```python
from build123d import *

# Parameters (mm, degrees)
SKETCH1_W           = 130
SKETCH1_H           = 180
BOSS_EXTRUDE1_DEPTH = 70
CUT_EXTRUDE1_DEPTH  = 131
FILLET2_R           = 4
SHELL1_T            = -2.5
SKETCH3_R           = 8
SKETCH3_W           = 60
SKETCH3_H           = 45
CUT_EXTRUDE2_DEPTH  = 10
CUT_EXTRUDE3_START  = -2.5
SKETCH4_W           = 69.3
SKETCH4_H           = 50
CUT_EXTRUDE3_DEPTH  = 1


with BuildPart() as part:
    # Sketch1 → Boss-Extrude1 (new body)
    with BuildSketch(Plane.XY):
        Rectangle(SKETCH1_W, SKETCH1_H)
    extrude(amount=BOSS_EXTRUDE1_DEPTH)

    # Sketch2 → Cut-Extrude1 (cut, through all)
    with BuildSketch(Plane.ZY.offset(65)):
        Polygon((70, -50), (25, -90), (70, -90), align=None)
    extrude(amount=-CUT_EXTRUDE1_DEPTH, mode=Mode.SUBTRACT)

    # Fillet2
    fillet2_edges = [part.edges().sort_by_distance(p)[0] for p in [
        (-65, 20, 70),
        (65, -90, 12.5),
        (-65, -90, 12.5),
        (0, -50, 70),
        (65, -70, 47.5),
        (0, -90, 25),
        (-65, -70, 47.5),
        (0, 90, 70),
        (65, 20, 70),
        (-65, 90, 35),
        (65, 90, 35),
    ]]
    fillet(fillet2_edges, radius=FILLET2_R)

    # Shell1
    shell1_openings = [part.faces().sort_by_distance(p)[0] for p in [
        (0, 0, 0),
    ]]
    offset(amount=SHELL1_T, openings=shell1_openings, kind=Kind.INTERSECTION)

    # Sketch3 → Cut-Extrude2 (cut)
    with BuildSketch(Plane(origin=(0, -62.689655172, 55.724137931), x_dir=(1, 0, 0), z_dir=(0, -0.747409319, 0.664363839))):
        with Locations((40.000108275, -9.586715238)):
            Circle(SKETCH3_R)
        with Locations((-11.005976929, -9.586715238)):
            Rectangle(SKETCH3_W, SKETCH3_H)
    extrude(amount=-CUT_EXTRUDE2_DEPTH, mode=Mode.SUBTRACT)

    # Sketch4 → Cut-Extrude3 (cut)
    with BuildSketch(Plane(origin=(0, -62.689655172, 55.724137931), x_dir=(1, 0, 0), z_dir=(0, -0.747409319, 0.664363839)).offset(CUT_EXTRUDE3_START)):
        with Locations((-8.85597671, -9.586715238)):
            Rectangle(SKETCH4_W, SKETCH4_H)
    extrude(amount=CUT_EXTRUDE3_DEPTH, mode=Mode.SUBTRACT)


solid = part.part
```
Geometry check sheet. Reference: the model listing, model coordinates, mm. A direction names the side the tool comes from. Coordinates: 2 decimals unless noted, no trailing zeros. Loops run counter-clockwise (first coordinate to the right, second up) from the corner with the lowest first, then second, coordinate; pieces in that order, holes last. Notation, with made-up numbers: (-30.75, 17.25) -> (-19.75, 17.25) arc R18 ccw to (-19.75, 44.25) -> close; hole circle Ø6 at (45, 84.5). An arc over 180 degrees is marked (long way). Put each result on its own line as item: value.
1) Cross-section at A-A on x = -13. Record the boundary of the cut face in (y, z), plus the area to 3 significant figures.
Result set:
outline: (-90, 0) -> (-87.5, 0) -> (-87.5, 23.48) arc R1.5 cw to (-87.12, 24.48) -> (-83.8, 28.21) -> (-84.55, 28.88) -> (-82.89, 30.75) -> (-84.01, 31.74) -> (-88.99, 26.14) arc R4 ccw to (-90, 23.48) -> close; (-54.11, 65.38) -> (-52.99, 64.38) -> (-51.33, 66.25) -> (-50.58, 65.58) -> (-49.32, 67) arc R1.5 cw to (-48.2, 67.5) -> (86, 67.5) arc R1.5 cw to (87.5, 66) -> (87.5, 0) -> (90, 0) -> (90, 66) arc R4 ccw to (86, 70) -> (-48.2, 70) arc R4 ccw to (-51.19, 68.66) -> close
area: 606 mm^2
2) Cross-section at B-B on y = -21. Record the boundary of the cut face in (x, z), plus the area to 3 significant figures.
Result set:
outline: (-65, 0) -> (-62.5, 0) -> (-62.5, 66) arc R1.5 cw to (-61, 67.5) -> (61, 67.5) arc R1.5 cw to (62.5, 66) -> (62.5, 0) -> (65, 0) -> (65, 66) arc R4 ccw to (61, 70) -> (-61, 70) arc R4 ccw to (-65, 66) -> close
area: 657 mm^2
3) Release check for a two-part mould opening along Y. For faces 3 (the flat face through (-1, 20, 70)), 4 (the cylindrical face through (0.854, 88.859, 68.797)), 5 (the flat face through (-43.506, -68, 47)) record: released by +Y, released by -Y, zero draft, split by the parting line, or undercut.
Result set:
face 3: zero draft
face 4: released by +Y
face 5: undercut
4) Tool access check on faces 1 (the flat face through (-1, -87.5, 12)), 2 (the cylindrical face through (-63.859, 19.838, 68.797)). Record the directions out of +Z, -Z, +X, -X, +Y, -Y that give a thin tool (end or side, any length) a straight path to the whole face; none if there is none.
Result set:
face 1: -Z
face 2: +Z, -X, +Y, -Y
5) Gauge pin test, flat ends, axial feed: pin 1 Ø10 at (y, z) = (-73.5, 49) entering from +X; pin 2 Ø1.5 at (x, z) = (37.5, 32) entering from -Y. Record the tip position at first contact, or that the pin passes through.
Result set:
pin 1: stops at x = 64.03
pin 2: stops at y = -84.44
6) Cross-section at C-C on z = 8.5. Record the boundary of the cut face in (x, y), plus the area to 3 significant figures.
Result set:
outline: (-65, -86) arc R4 ccw to (-61, -90) -> (61, -90) arc R4 ccw to (65, -86) -> (65, 86) arc R4 ccw to (61, 90) -> (-61, 90) arc R4 ccw to (-65, 86) -> close; hole (-62.5, -86) arc R1.5 ccw to (-61, -87.5) -> (61, -87.5) arc R1.5 ccw to (62.5, -86) -> (62.5, 86) arc R1.5 ccw to (61, 87.5) -> (-61, 87.5) arc R1.5 ccw to (-62.5, 86) -> close
area: 1,510 mm^2
7) Thickness scan on line 1 (X direction, y = -9.5, z = 15); line 2 (Y direction, x = -6, z = 17.5); line 3 (Z direction, x = 9.5, y = 28). Record the ranges inside material, lowest first.
Result set:
line 1: x = -65 to -62.5, 62.5 to 65
line 2: y = -90 to -87.5, 87.5 to 90
line 3: z = 67.5 to 70
8) Cross-section at D-D on x = -52. Record the boundary of the cut face in (y, z), plus the area to 3 significant figures.
Result set:
outline: (-90, 0) -> (-87.5, 0) -> (-87.5, 23.48) arc R1.5 cw to (-87.12, 24.48) -> (-49.32, 67) arc R1.5 cw to (-48.2, 67.5) -> (86, 67.5) arc R1.5 cw to (87.5, 66) -> (87.5, 0) -> (90, 0) -> (90, 66) arc R4 ccw to (86, 70) -> (-48.2, 70) arc R4 ccw to (-51.19, 68.66) -> (-88.99, 26.14) arc R4 ccw to (-90, 23.48) -> close
area: 723 mm^2
